Input: dimensioned drawing with shaded views. Units: mm. Origin: part minimum x, y, z. A direction names the side the tool comes from. Give positions to 0.01 mm unless a question says otherwise; leave off trailing zeros. Write each loop counter-clockwise with the first axis right and the second up, starting at its lowest first coordinate (ties: lowest second). Pieces come first, ordered by that corner, then holes. Notation, with made-up numbers: (-6.75, 88) -> (2.25, 88) arc R20 cw to (2.25, 102) -> close; hole circle Ø4 at (36.5, 75). An arc over 180 degrees is marked (long way). Return JSON: item names as keys, results as strings. Group by question number.
Item 1: Line query: line 1 (Y direction, x = 144.5, z = 144.5); line 2 (Y direction, x = 555, z = 33); line 3 (X direction, y = 12.5, z = 128). Output: solid intervals per line, ascending. Write a range as [from, to].
Item 2: Section D-D, the plane x = 606. Return loops of the section in (y, z).
Item 3: Mould query, pull axis X, two halves, no side actions, for the marked faces 1, 2 and 3. Classes: released by +X, released by -X, zero draft, split by the parting line, or undercut.
Item 4: Pin query (flat end, axial travel): P1, Ø2, axis at y = 39, z = 173, coming from the +X side (1 decimal); P2, Ø10, axis at y = 22.5, z = 46.5, coming from the +X side; P3, Ø5, axis at y = 18.5, z = 222.5, coming from the +X side. Return the tip coordinate at first contact, or that it passes through.
Item 5: Section C-C, the plane x = 756. Return loops of the section in (y, z), then the cut area to 3 significant figures.
Item 6: Section A-A, the plane y = 34.5. Return loops of the section in (x, z) (1 decimal), then the cut area to 3 significant figures.
Item 7: Set-up query: the marked faces 4, 5, 6 and 7. Return all of +Z, -Z, +X, -X, +Y, -Y with unobstructed straight access to the full face (end or side cutting, diameter ignored); none if empty.
Item 8: Section B-B, the plane z = 27.5. Return loops of the section in (x, y) (1 decimal), then the cut area to 3 significant figures.
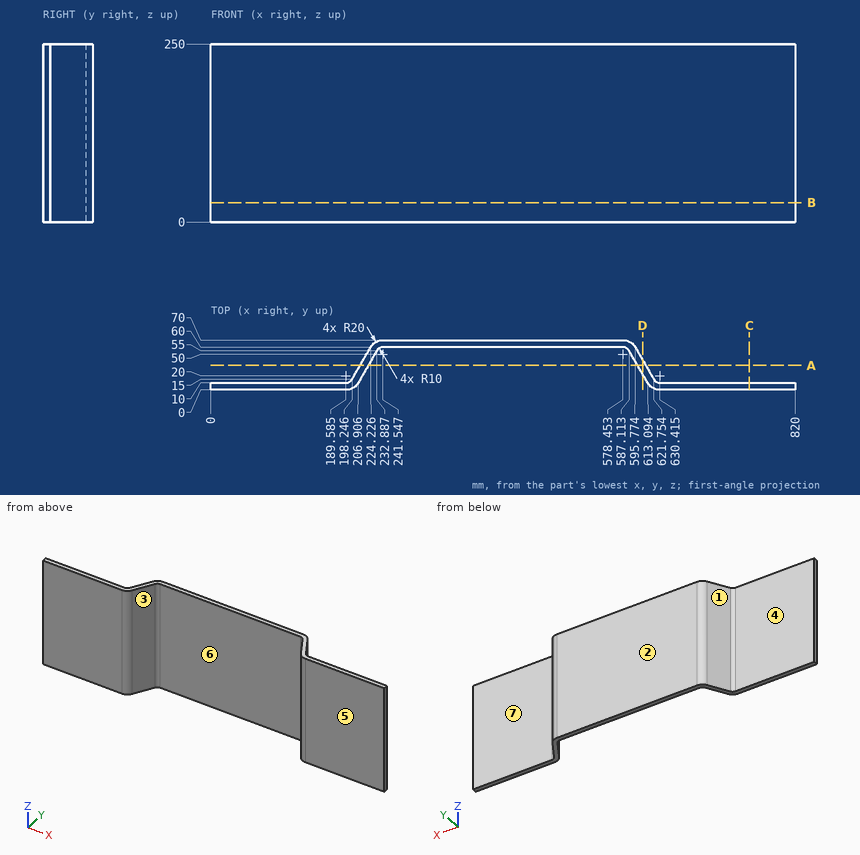
Answer below:
{
 "1": {"line 1": "y = [0, 10]", "line 2": "y = [60, 70]", "line 3": "x = [196.2, 208.35], [611.65, 623.8]"},
 "2": {"outline": "(22.29, 0) -> (42.29, 0) -> (42.29, 250) -> (22.29, 250) -> close"},
 "3": {"face 1": "released by -X", "face 2": "zero draft", "face 3": "undercut"},
 "4": {"P1": "stops at x = 608.5", "P2": "stops at x = 620.31", "P3": "stops at x = 621.18"},
 "5": {"outline": "(0, 0) -> (10, 0) -> (10, 250) -> (0, 250) -> close", "area": "2,500 mm2"},
 "6": {"outline": "(209.5, 0) -> (221.1, 0) -> (221.1, 250) -> (209.5, 250) -> close; (598.9, 0) -> (610.5, 0) -> (610.5, 250) -> (598.9, 250) -> close", "area": "5,770 mm2"},
 "7": {"face 4": "+Z, -Z, -X, +Y", "face 5": "+Z, -Z, +X, -X, -Y", "face 6": "+Z, -Z, -Y", "face 7": "+Z, -Z, +X, +Y"},
 "8": {"outline": "(0, 0) -> (189.6, 0) arc R20 ccw to (206.9, 10) -> (232.9, 55) arc R10 cw to (241.5, 60) -> (578.5, 60) arc R10 cw to (587.1, 55) -> (613.1, 10) arc R20 ccw to (630.4, 0) -> (820, 0) -> (820, 10) -> (630.4, 10) arc R10 cw to (621.8, 15) -> (595.8, 60) arc R20 ccw to (578.5, 70) -> (241.5, 70) arc R20 ccw to (224.2, 60) -> (198.2, 15) arc R10 cw to (189.6, 10) -> (0, 10) -> close", "area": "8,830 mm2"}
}
